Can you work these out from the model? Positions are in its coordinate system, mm. Face numbers are marked on the shaded views. A direction names the side the tool comes from. Round coordinates to 2 decimals unless told otherwise and drop trailing zeros. Loops run counter-clockwise (first coordinate to the right, second up) from the corner with the lowest first, then second, coordinate; pieces in that order, holes last.
Autodesk Inventor part; units mm, degrees
ref_plane "part1_to_part2_XY" through (5, 0, 0) normal (1, 0, 0) x (0, 0, -1)
ref_plane "part1_to_part2_YZ" through (5, 0, 0) normal (0, 0, -1) x (0, 1, 0)
ref_plane "part1_to_part2_ZX" through (5, 0, 0) normal (0, 1, 0) x (1, 0, 0)
sketch "Sketch_1" plane through (0, 0, 0) normal (0, 0, 1) x (1, 0, 0)
  line L0 (5, 0) -> (-5, 0)
  line L1 (-5, 0) -> (-5, 23.5)
  line L2 (-5, 23.5) -> (-2.8868, 23.5)
  line L3 (-2.8868, 23.5) -> (-1.7321, 21.5)
  arc A0 (-1.7321, 21.5) -> (1.7321, 21.5) centre (0, 22.5) ccw
  line L4 (1.7321, 21.5) -> (2.8868, 23.5)
  line L5 (2.8868, 23.5) -> (5, 23.5)
  line L6 (5, 23.5) -> (5, 0)
  line L7 (5, 0) -> (-5, 0)
revolve "Revolution1" add sketch "Sketch_1" angle 360 about axis through (5, 0, 0) along (1, 0, 0)
sketch "Sketch_2" plane through (0, 0, 0) normal (0, 0, 1) x (1, 0, 0)
  line L0 (5, 0) -> (15, 0)
  line L1 (15, 0) -> (15, -12)
  line L2 (15, -12) -> (14.5, -12.5)
  line L3 (14.5, -12.5) -> (5, -12.5)
  line L4 (5, -12.5) -> (5, 0)
  line L5 (5, 0) -> (15, 0)
revolve "Revolution2" add sketch "Sketch_2" angle 180 mid plane about axis through (5, 0, 0) along (1, 0, 0)
sketch "Sketch_3" plane through (0, 0, 0) normal (0, 0, 1) x (1, 0, 0)
  line L0 (5, -0.5) -> (15, -0.5)
  line L1 (15, -0.5) -> (15, 0)
  line L2 (15, 0) -> (5, 0)
  line L3 (5, 0) -> (5, -0.5)
extrude "Extrusion1" cut sketch "Sketch_3" along normal mid plane 50
sketch "Sketch_4" plane through (0, 0, 0) normal (0, 0, 1) x (1, 0, 0)
  line L0 (15, 0) -> (-5, 0)
  line L1 (-5, 0) -> (-5, 5)
  line L2 (-5, 5) -> (15, 5)
  line L3 (15, 5) -> (15, 0)
  line L4 (15, 0) -> (-5, 0)
revolve "Revolution3" cut sketch "Sketch_4" angle 360 about axis through (15, 0, 0) along (1, 0, 0)
sketch "Sketch_5" plane through (0, 0, 9) normal (0, 0, 1) x (1, 0, 0)
  line L0 (10.5, -12.5) -> (10.5, -0.5)
  line L1 (10.5, -0.5) -> (12.5, -0.5)
  line L2 (12.5, -0.5) -> (12.121, -0.879)
  line L3 (12.121, -0.879) -> (12.121, -12.121)
  line L4 (12.121, -12.121) -> (12.5, -12.5)
  line L5 (12.5, -12.5) -> (10.5, -12.5)
  line L6 (10.5, -12.5) -> (10.5, -0.5)
revolve "Revolution4" cut sketch "Sketch_5" angle 360 about axis through (10.5, -12.5, 9) along (0, -1, 0)
thread "Thread1"
sketch "Sketch_6" plane through (0, 0, -9) normal (0, 0, 1) x (1, 0, 0)
  line L0 (10.5, -12.5) -> (10.5, -0.5)
  line L1 (10.5, -0.5) -> (12.5, -0.5)
  line L2 (12.5, -0.5) -> (12.121, -0.879)
  line L3 (12.121, -0.879) -> (12.121, -12.121)
  line L4 (12.121, -12.121) -> (12.5, -12.5)
  line L5 (12.5, -12.5) -> (10.5, -12.5)
  line L6 (10.5, -12.5) -> (10.5, -0.5)
revolve "Revolution5" cut sketch "Sketch_6" angle 360 about axis through (10.5, -12.5, -9) along (0, -1, 0)
thread "Thread2"
ref_plane "part1_to_part2_XY" through (5, 0, 0) normal (1, 0, 0) x (0, 0, -1)
ref_plane "part1_to_part2_YZ" through (5, 0, 0) normal (0, 0, -1) x (0, 1, 0)
ref_plane "part1_to_part2_ZX" through (5, 0, 0) normal (0, 1, 0) x (1, 0, 0)
properties part number "MBRAC45-2-10p1"
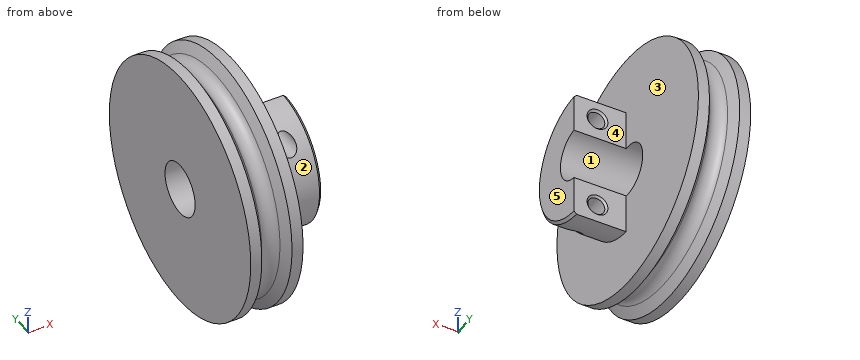
(1) Suppose I cut it at C-C (x = 1). Write out the boundary of the cut face in (y, z).
(2) We'd pull the mould along Z, two halves only. Please class the marked faces 1, 2 and 3: released by +Z, released by -Z, zero draft, split by the parting line, or undercut.
(3) If I drill on line 1 (X direction, y = -4, z = -9); line 2 (Z direction, x = 10.5, y = -4.25); line 3 (X direction, y = 5, z = 14), over which ranges is the centre line in solid material (lowest first)?
(4) Suppose I cut it at B-B (x = 10.5). Write out the boundary of the cut face in (y, z).
(5) For pin 1 (5 mm diameter, centred on y = 8.5, z = 14.5, fed in from +X); pin 2 (1 mm diameter, centred on x = -1, y = -13, fed in from +Z); pin 3 (16 mm diameter, centred on y = 0, z = 0, fed in from -X); pin 4 (4 mm diameter, centred on x = 9.5, z = 8.5, fed in from +Y), each with a flat end and sliding along its axis, tell me the tip position at first contact or that it passes through.
(6) Suppose I cut it at A-A (z = 0). Write out the boundary of the cut face in (x, y).
(7) Which directions (+Z, -Z, +X, -X, +Y, -Y) give clear straight access to the entire face, cutting with the end or side of a thin tool? Please do the marked faces 4 and 5.
Check result:
1. outline: circle Ø41.54 at (0, 0); hole circle Ø10 at (0, 0)
2. face 1: undercut
2. face 2: split by the parting line
2. face 3: zero draft
3. line 1: x = -5 to 8.88, 12.12 to 15
3. line 2: z = -11.76 to -10.62, -7.38 to -2.63, 2.63 to 7.38, 10.62 to 11.76
3. line 3: x = -5 to 5
4. outline: (-10.09, -7.38) - (-0.88, -7.38) - (-0.5, -7) - (-0.5, -4.97) arc R5 cw to (-0.5, 4.97) - (-0.5, 7) - (-0.88, 7.38) - (-10.09, 7.38) arc R12.5 ccw to start; (-6.59, -10.62) arc R12.5 ccw to (-0.5, -12.49) - (-0.5, -11) - (-0.88, -10.62) - close; (-6.59, 10.62) - (-0.88, 10.62) - (-0.5, 11) - (-0.5, 12.49) arc R12.5 ccw to start
5. pin 1: stops at x = 5
5. pin 2: stops at z = 16.82
5. pin 3: stops at x = -5
5. pin 4: stops at y = -0.5
6. outline: (-5, -23.5) - (-2.89, -23.5) - (-1.73, -21.5) arc R2 cw to (1.73, -21.5) - (2.89, -23.5) - (5, -23.5) - (5, -12.5) - (14.5, -12.5) - (15, -12) - (15, -5) - (-5, -5) - close; (-5, 5) - (5, 5) - (5, 23.5) - (2.89, 23.5) - (1.73, 21.5) arc R2 cw to (-1.73, 21.5) - (-2.89, 23.5) - (-5, 23.5) - close
7. face 4: +Z, -Z, +X, +Y
7. face 5: +Z, -Z, +X, +Y, -Y
